Could you check a few things on this model? Use its own coordinates, in mm. Give positions to 0.01 mm unless a question says otherwise; leave off trailing zeros. Order: outer loops, then holes, each group sorted by start corner. A loop starts at its lowest first (then second) coordinate and runs counter-clockwise, first axis right, second up. Notation, with made-up numbers: (-30, 64) - (15, 64) arc R21 ccw to (15, 86) - close; hole circle Ø11 at (7.5, -4.75). An arc over 180 degrees is marked (long way). Put each result on its own line as item: value.
Autodesk Inventor part; units mm, degrees
ref_plane "YZ Plane" through (0, 0, 0) normal (1, 0, 0) x (0, 1, 0)
ref_plane "XZ Plane" through (0, 0, 0) normal (0, 1, 0) x (-1, 0, 0)
ref_plane "XY Plane" through (0, 0, 0) normal (0, 0, 1) x (1, 0, 0)
sketch "Sketch1" plane through (0, 0, 0) normal (0, 1, 0) x (-1, 0, 0)
  line L0 (-21, 29) -> (21, 29)
  line L1 (21, 29) -> (21, -29)
  line L2 (21, -29) -> (-21, -29)
  line L3 (-21, -29) -> (-21, 29)
  line L4 (-21, 29) -> (21, -29) construction
  line L5 (21, 29) -> (-21, -29) construction
  point P0 (0, 0)
  dimension "d0" = 42
  dimension "d1" = 58
extrude "Extrusion1" add sketch "Sketch1" along normal blind 1
sketch "Sketch4" plane through (0, 0, 0) normal (0, -1, 0) x (1, 0, 0)
  line L0 (-21, 29) -> (21, 29)
  line L1 (21, 29) -> (18.5, 29)
  line L2 (18.5, 29) -> (18.5, 26.5)
  line L3 (18.5, 26.5) -> (21, 26.5)
  line L4 (21, 26.5) -> (21, 29)
  circle A0 centre (18.5, 26.5) radius 1.25
  point P0 (0, 0)
  dimension "d42" = 2.5
  dimension "d43" = 2.5
  dimension "d44" = 2.5
extrude "Extrusion2" cut sketch "Sketch4" against normal through all contours A0 L3 L2 | L2 L3 A0
sketch "Sketch5" plane through (0, 0, 0) normal (0, -1, 0) x (1, 0, 0)
  line L0 (-21, -29) -> (21, -29)
  line L1 (-21, -29) -> (-18.5, -29)
  line L2 (-18.5, -29) -> (-18.5, -26.5)
  line L3 (-18.5, -26.5) -> (-21, -26.5)
  line L4 (-21, -26.5) -> (-21, -29)
  circle A0 centre (-18.5, -26.5) radius 1.25
  point P0 (0, 0)
  dimension "d49" = 2.5
  dimension "d50" = 2.5
  dimension "d51" = 2.5
extrude "Extrusion3" cut sketch "Sketch5" against normal through all contours A0 L3 L2 | L2 L3 A0
sketch "Sketch6" plane through (0, 1, 0) normal (0, 1, 0) x (1, 0, 0)
  line L0 (-21, -29) -> (21, -29)
  line L1 (-21, -29) -> (-18.5, -29)
  line L2 (-18.5, -29) -> (-18.5, -26.5)
  line L3 (-18.5, -26.5) -> (-21, -26.5)
  line L4 (-21, -26.5) -> (-21, -29)
  circle A0 centre (-18.5, -26.5) radius 1.25
  point P0 (0, 0)
  dimension "d60" = 2.5
  dimension "d61" = 2.5
  dimension "d62" = 2.5
extrude "Extrusion4" cut sketch "Sketch6" against normal up to next contours A0 L3 L2 | L2 L3 A0
sketch "Sketch7" plane through (0, 0, 0) normal (0, -1, 0) x (1, 0, 0)
  circle A0 centre (18.5, -26.5) radius 1.25
  line L0 (-21, -29) -> (21, -29)
  line L1 (21, -29) -> (21, 29)
  point P0 (0, 0)
  dimension "d67" = 2.5
  dimension "d68" = 2.5
  dimension "d69" = 2.5
extrude "Extrusion5" cut sketch "Sketch7" against normal up to next
properties part number "regulator"
1) I'm going to push a flat-ended pin straight in: pin 1 (1.5 mm diameter, centred on x = 18.5, z = 26.5, fed in from +Y). Where does the tip first touch, or does it pass through?
Filled in:
pin 1: passes through
2) Suppose I cut it at A-A, the plane x = 18.5. List the corners of the cut face in (y, z) for me.
Filled in:
outline: (0, -29) - (1, -29) - (1, -27.75) - (0, -27.75) - close; (0, -25.25) - (1, -25.25) - (1, 25.25) - (0, 25.25) - close; (0, 27.75) - (1, 27.75) - (1, 29) - (0, 29) - close
3) Suppose I cut it at B-B, the plane z = -26.5. List the corners of the cut face in (x, y) for me.
Filled in:
outline: (-21, 0) - (-19.75, 0) - (-19.75, 1) - (-21, 1) - close; (-17.25, 0) - (17.25, 0) - (17.25, 1) - (-17.25, 1) - close; (19.75, 0) - (21, 0) - (21, 1) - (19.75, 1) - close
4) We'd pull the mould along Z, two halves only. Please class faces 1 (the flat face through (0, 1, 0)), 2 (the cylindrical face through (19.655, 0.493, -26.979)): pulls with the +Z half, pulls with the -Z half, needs draft (parallel to the pull), parting line crosses it, or undercut.
Filled in:
face 1: needs draft
face 2: undercut
5) If I drill on line 1 (Z direction, x = -18.5, y = 0.45); line 2 (X direction, y = 0.55, z = 26), over which ranges is the centre line in solid material (lowest first)? Write a range as [from, to].
Filled in:
line 1: z = [-29, -27.75], [-25.25, 25.25], [27.75, 29]
line 2: x = [-21, -19.65], [-17.35, 17.35], [19.65, 21]
